Verification items for this drawing (mm, ordinates from the low corner). Coordinates: 2 decimals unless noted, no trailing zeros. Order: outer loops, then holes, each group sorted by start corner. A loop starts at its lowest first (then second) coordinate and runs counter-clockwise, first axis right, second up. Notation, with made-up numbers: (84.5, 10.25) -> (90.5, 10.25) arc R24 cw to (90.5, 28.25) -> close; hole circle Ø1 at (63, 42.5). An arc over 180 degrees is marked (long way). Write item = value, one per line. Start each with the question number.
1. Cross-section at A-A on z = 65. Record the cut outline in (x, y) (3 decimals).
2. Cross-section at B-B on y = 0.75. Record the cut outline in (x, z).
3. Cross-section at C-C on x = 3. Record the cut outline in (y, z) (3 decimals).
4. Thickness scan on line 1 along X through (y, z) = (0.9, 65); line 2 along Z through (x, y) = (21, 2.45). Record the ranges inside material, lowest first. Write a range as from..to.
5. Go/stop test with flat-tipped pins: P1, Ø1.6, axis at y = 1, z = 66, coming from the +X side; P2, Ø1, axis at x = 24, y = 2, coming from the +Z side; P3, Ø1.5, axis at x = 19, z = 61, coming from the -Y side; P4, Ø1.6, axis at y = 1.5, z = 66, coming from the -X side. Record where each tip stops, or that it passes through.
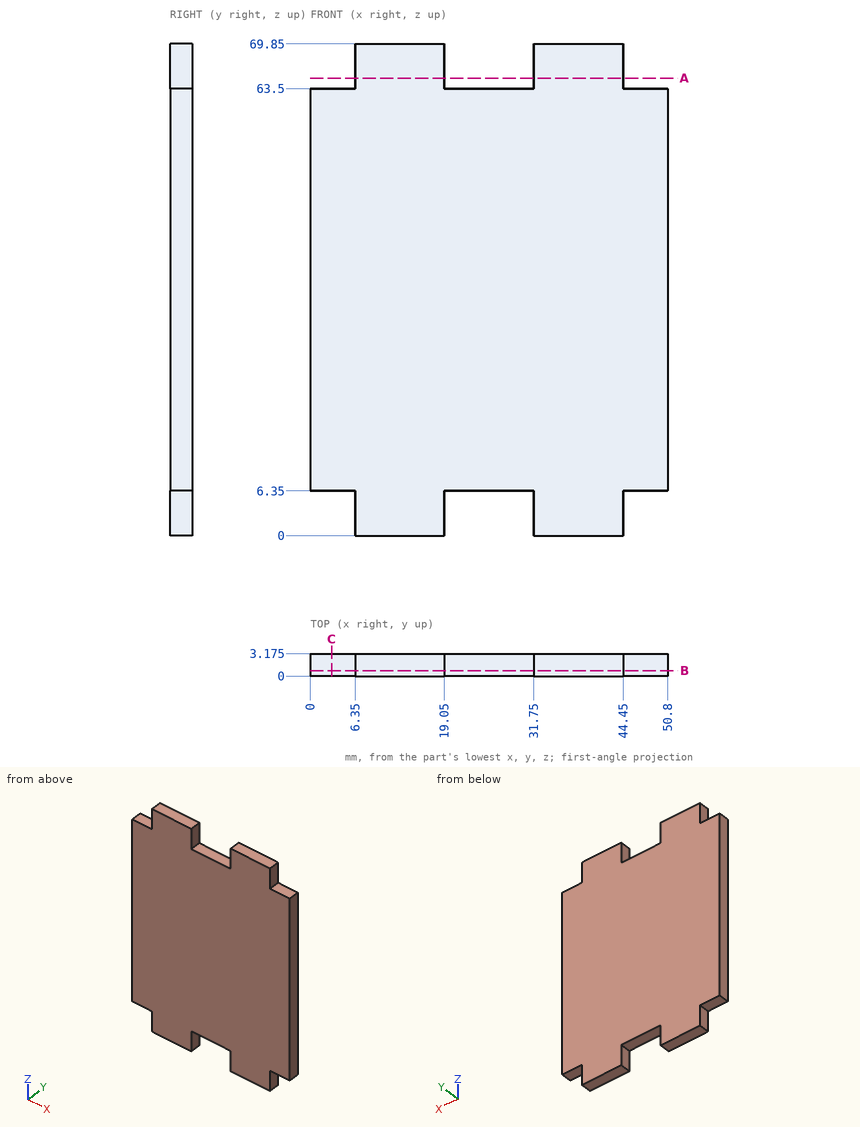
Worked out:
q1.outline = (6.35, 0) -> (19.05, 0) -> (19.05, 3.175) -> (6.35, 3.175) -> close; (31.75, 0) -> (44.45, 0) -> (44.45, 3.175) -> (31.75, 3.175) -> close
q2.outline = (0, 6.35) -> (6.35, 6.35) -> (6.35, 0) -> (19.05, 0) -> (19.05, 6.35) -> (31.75, 6.35) -> (31.75, 0) -> (44.45, 0) -> (44.45, 6.35) -> (50.8, 6.35) -> (50.8, 63.5) -> (44.45, 63.5) -> (44.45, 69.85) -> (31.75, 69.85) -> (31.75, 63.5) -> (19.05, 63.5) -> (19.05, 69.85) -> (6.35, 69.85) -> (6.35, 63.5) -> (0, 63.5) -> close
q3.outline = (0, 6.35) -> (3.175, 6.35) -> (3.175, 63.5) -> (0, 63.5) -> close
q4.line_1 = 6.35..19.05, 31.75..44.45
q4.line_2 = 6.35..63.5
q5.P1 = 44.45
q5.P2 = 63.5
q5.P3 = 0
q5.P4 = 6.35
